Could you check a few things on this model? Use its own coordinates, in mm. A direction names the side the tool comes from. Round coordinates to 2 decimals unless told otherwise and drop trailing zeros. Loops run counter-clockwise (first coordinate to the right, second up) from the corner with the lowest first, then second, coordinate; pieces in that order, holes last.
from build123d import *

# Parameters (mm, degrees)
F0_W          = 100
F0_H          = 150
F1_DEPTH      = 3
F2_R          = 1.5
F3_DEPTH      = 40
F3_TAPER      = -0.8
F4_W          = 1.5
F4_H          = 1.5
F5_DEPTH      = 23
F5_TAPER      = -0.5
F6_W          = 22.2306074575
F6_H          = 11.5619013086
F7_DEPTH      = 4.6
F7_DEPTH_BACK = 0.4
F9_DEPTH      = 3
F10_W         = 1.5
F10_H         = 65
F10_H_2       = 23
F11_DEPTH     = 15
F12_W         = 1.28
F12_H         = 13
F12_W_2       = 1.2995073211
F13_DEPTH     = 2


with BuildPart() as f1:
    # F0 (on Top) → F1 (new body)
    with BuildSketch(Plane.XY):
        with Locations((1.3026602566, 11.9441717863)):
            Rectangle(F0_W, F0_H)
    extrude(amount=F1_DEPTH)

    # F2 (on face) → F3 (join)
    with BuildSketch(Plane.XY.offset(3)):
        with Locations((0, 60.0040182471)):
            Circle(F2_R)
        with Locations((-24.9959174544, 0)):
            Circle(F2_R)
        with Locations((24.9958131462, 0)):
            Circle(F2_R)
    extrude(amount=F3_DEPTH, taper=F3_TAPER)

    # F4 (on face) → F5 (join)
    with BuildSketch(Plane.XY.offset(3)):
        with Locations((-10.6072969437, -12.6336732581)):
            Rectangle(F4_W, F4_H)
        with Locations((9.6686085388, -12.6336732581)):
            Rectangle(F4_W, F4_H)
        with Locations((-10.6072969437, -22.2625773102)):
            Rectangle(F4_W, F4_H)
        with Locations((9.6686085388, -22.2625773102)):
            Rectangle(F4_W, F4_H)
    extrude(amount=F5_DEPTH, taper=F5_TAPER)

    # F6 (on face) → F7 (join, two sides)
    with BuildSketch(Plane.XY.offset(26)) as f7_sk:
        with Locations((-0.4788641818, -17.4084207974)):
            Rectangle(F6_W, F6_H)
    extrude(amount=F7_DEPTH)
    extrude(f7_sk.sketch, amount=-F7_DEPTH_BACK)

    # F8 (on face) → F9 (join)
    with BuildSketch(Plane.XY.offset(43)):
        with BuildLine():
            Line((-36.0795073211, 57.7763375454), (-36.0795073211, -7.2236624546))
            Line((-36.0795073211, -7.2236624546), (33.9204926789, -7.2236624546))
            Line((33.9204926789, -7.2236624546), (33.9204926789, 15.7763375454))
            ThreePointArc((33.9204926789, 15.7763375454), (29.5270943967, 26.3829392632), (18.9204926789, 30.7763375454))
            ThreePointArc((18.9204926789, 30.7763375454), (8.3138909611, 35.1697358276), (3.9204926789, 45.7763375454))
            Line((3.9204926789, 45.7763375454), (3.9204926789, 57.7763375454))
            ThreePointArc((3.9204926789, 57.7763375454), (-0.4729056033, 68.3829392632), (-11.0795073211, 72.7763375454))
            Line((-11.0795073211, 72.7763375454), (-21.0795073211, 72.7763375454))
            ThreePointArc((-21.0795073211, 72.7763375454), (-31.6861090389, 68.3829392632), (-36.0795073211, 57.7763375454))
        make_face()
    extrude(amount=F9_DEPTH)

    # F10 (on face) → F11 (join)
    with BuildSketch(Plane.XY.offset(46)):
        with Locations((-35.3295073211, 25.2763375454)):
            Rectangle(F10_W, F10_H)
        with Locations((33.1704926789, 4.2763375454)):
            Rectangle(F10_W, F10_H_2)
    extrude(amount=F11_DEPTH)

    # F12 (on face) → F13 (join)
    with BuildSketch(Plane.XY.offset(46)):
        with Locations((-33.9395073211, 6.5)):
            Rectangle(F12_W, F12_H)
        with Locations((-32.6595073211, 6.5)):
            Rectangle(F12_W, F12_H)
        with Locations((-31.3795073211, 6.5)):
            Rectangle(F12_W, F12_H)
        with Locations((-30.0995073211, 6.5)):
            Rectangle(F12_W, F12_H)
        with Locations((-28.8195073211, 6.5)):
            Rectangle(F12_W, F12_H)
        with Locations((-27.5395073211, 6.5)):
            Rectangle(F12_W, F12_H)
        with Locations((-26.2595073211, 6.5)):
            Rectangle(F12_W, F12_H)
        with Locations((-24.9795073211, 6.5)):
            Rectangle(F12_W, F12_H)
        with Locations((-23.6995073211, 6.5)):
            Rectangle(F12_W, F12_H)
        with Locations((-22.4195073211, 6.5)):
            Rectangle(F12_W, F12_H)
        with Locations((-21.1395073211, 6.5)):
            Rectangle(F12_W, F12_H)
        with Locations((-19.8595073211, 6.5)):
            Rectangle(F12_W, F12_H)
        with Locations((-18.5795073211, 6.5)):
            Rectangle(F12_W, F12_H)
        with Locations((-17.2995073211, 6.5)):
            Rectangle(F12_W, F12_H)
        with Locations((-16.0195073211, 6.5)):
            Rectangle(F12_W, F12_H)
        with Locations((-14.7395073211, 6.5)):
            Rectangle(F12_W, F12_H)
        with Locations((-13.4595073211, 6.5)):
            Rectangle(F12_W, F12_H)
        with Locations((-12.1795073211, 6.5)):
            Rectangle(F12_W, F12_H)
        with Locations((-10.8995073211, 6.5)):
            Rectangle(F12_W, F12_H)
        with Locations((-9.6195073211, 6.5)):
            Rectangle(F12_W, F12_H)
        with Locations((-8.3395073211, 6.5)):
            Rectangle(F12_W, F12_H)
        with Locations((-7.0595073211, 6.5)):
            Rectangle(F12_W, F12_H)
        with Locations((-5.7795073211, 6.5)):
            Rectangle(F12_W, F12_H)
        with Locations((-4.4995073211, 6.5)):
            Rectangle(F12_W, F12_H)
        Polygon((-3.8595073211, 13), (-3.8595073211, 0), (-3.8595073211, -0.0326875597), (-2.5795073211, -0.0326875597), (-2.5795073211, 13), align=None)
        Polygon((-1.2995073211, 13), (-2.5795073211, 13), (-2.5795073211, -0.0326875597), (-1.2995073211, -0.0326875597), (-1.2995073211, 0), align=None)
        with Locations((-0.6497536606, 6.5)):
            Rectangle(F12_W_2, F12_H)
    extrude(amount=F13_DEPTH)


solid = f1.part
Item 1: If we section it at B-B, the plane x = 15.5: Please give me the cut outline in (y, z).
Results list:
outline: (-63.06, 0) - (86.94, 0) - (86.94, 3) - (-63.06, 3) - close; (-7.22, 43) - (31.17, 43) - (31.17, 46) - (-7.22, 46) - close
Item 2: Will these pins go through, and if not, where does the flat tip stop? pin 1 (10 mm diameter, centred on x = 27.5, z = 19, fed in from +Y); pin 2 (6 mm diameter, centred on x = 3.5, y = -18, fed in from +Z); pin 3 (2.5 mm diameter, centred on x = -18, z = 44.5, fed in from +Y); pin 4 (1 mm diameter, centred on y = -9.5, z = 26, fed in from +X).
Results list:
pin 1: stops at y = 1.78
pin 2: stops at z = 30.6
pin 3: stops at y = 72.78
pin 4: passes through
Item 3: If we section it at A-A, the plane y = 10: Please give me the cut outline in (x, z), then the cut area to 3 significant figures.
Results list:
outline: (-48.7, 0) - (51.3, 0) - (51.3, 3) - (-48.7, 3) - close; (-36.08, 43) - (33.92, 43) - (33.92, 61) - (32.42, 61) - (32.42, 46) - (0, 46) - (0, 48) - (-34.58, 48) - (-34.58, 61) - (-36.08, 61) - close
area: 624 mm2
Item 4: For faces 4 (the flat face through (33.92, 4, 52)), 5 (the flat face through (-36.08, 25, 52)), 6 (the flat face through (32.42, 4, 53)), 7 (the conical face through (-0.232, 61.772, 23.28)), which set-ups out of +Z, -Z, +X, -X, +Y, -Y let a thin tool reach every point of the face, with its end or its side?
Results list:
face 4: +Z, +X, +Y, -Y
face 5: +Z, -X, +Y, -Y
face 6: +Z, +Y, -Y
face 7: none
Item 5: If we section it at C-C, the plane z = 40.5: Please give me the cut outline in (x, y).
Results list:
outline: circle Ø4.05 at (-25, 0); circle Ø4.05 at (0, 60); circle Ø4.05 at (25, 0)
Item 6: We'd pull the mould along Y, two halves only. Please class faces 1 (the flat face through (-1, -17, 25.6)), 2 (the flat face through (1, 86.944, 1)), 3 (the flat face through (10.636, -17, 28)): released by +Y, released by -Y, zero draft, split by the parting line, or undercut.
Results list:
face 1: undercut
face 2: released by +Y
face 3: zero draft
Item 7: If we section it at D-D, the plane y = 66: Please give me the cut outline in (x, z), then the cut area to 3 significant figures.
Results list:
outline: (-48.7, 0) - (51.3, 0) - (51.3, 3) - (-48.7, 3) - close; (-33.62, 43) - (1.47, 43) - (1.47, 46) - (-33.62, 46) - close
area: 405 mm2
Item 8: If I drill on line 1 along Z through (x, y) = (-31.5, 55); line 2 along Z through (x, y) = (-30.5, 9.5); line 3 along Z through (x, y) = (37, 53), over which ranges is the centre line in solid material (lowest first)?
Results list:
line 1: z = 0 to 3, 43 to 46
line 2: z = 0 to 3, 43 to 48
line 3: z = 0 to 3
